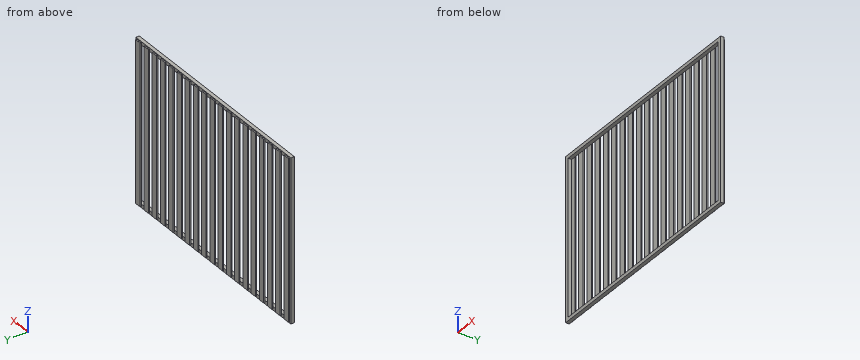
from build123d import *

# Parameters (mm, degrees)
F0_W     = 1900
F0_H     = 1400
F0_W_2   = 1840
F0_H_2   = 1340
F1_DEPTH = 15
F2_W     = 55
F2_H     = 10
F3_DEPTH = 690


# Not quite as in the source:
# - a feature names something its author has since deleted; it is built from what else it names


with BuildPart() as f1:
    # F0 (on Front) → F1 (new body, symmetric)
    with BuildSketch(Plane.XZ):
        Rectangle(F0_W, F0_H)
        Rectangle(F0_W_2, F0_H_2, mode=Mode.SUBTRACT)
    extrude(amount=F1_DEPTH, both=True)

    # F2 (on Top) → F3 (join, symmetric)
    with BuildSketch(Plane.XY):
        with Locations((-907.5, 20)):
            Rectangle(F2_W, F2_H)
        with Locations((-806.5, 20)):
            Rectangle(F2_W, F2_H)
        with Locations((-705.5, 20)):
            Rectangle(F2_W, F2_H)
        with Locations((-604.5, 20)):
            Rectangle(F2_W, F2_H)
        with Locations((-503.5, 20)):
            Rectangle(F2_W, F2_H)
        with Locations((-402.5, 20)):
            Rectangle(F2_W, F2_H)
        with Locations((-301.5, 20)):
            Rectangle(F2_W, F2_H)
        with Locations((-200.5, 20)):
            Rectangle(F2_W, F2_H)
        with Locations((-99.5, 20)):
            Rectangle(F2_W, F2_H)
        with Locations((1.5, 20)):
            Rectangle(F2_W, F2_H)
        with Locations((102.5, 20)):
            Rectangle(F2_W, F2_H)
        with Locations((203.5, 20)):
            Rectangle(F2_W, F2_H)
        with Locations((304.5, 20)):
            Rectangle(F2_W, F2_H)
        with Locations((405.5, 20)):
            Rectangle(F2_W, F2_H)
        with Locations((506.5, 20)):
            Rectangle(F2_W, F2_H)
        with Locations((607.5, 20)):
            Rectangle(F2_W, F2_H)
        with Locations((708.5, 20)):
            Rectangle(F2_W, F2_H)
        with Locations((809.5, 20)):
            Rectangle(F2_W, F2_H)
        with Locations((910.5, 20)):
            Rectangle(F2_W, F2_H)
    extrude(amount=F3_DEPTH, both=True)


solid = f1.part
Build history of the part. All positions in model axes, mm. Round coordinates to 2 decimals unless told otherwise and drop trailing zeros. Write each loop counter-clockwise with the first axis right and the second up, starting at its lowest first coordinate (ties: lowest second). Pieces come first, ordered by that corner, then holes. Notation, with made-up numbers: (43, 56.25) -> (53, 56.25) arc R24 ccw to (53, 88.25) -> close; hole circle Ø1 at (46, -13). An arc over 180 degrees is marked (long way). Write item = value, one per line.
(1) Flat gauge pins, fed straight in: pin 1 (3 mm diameter, centred on y = 22.5, z = -91, fed in from -X); pin 2 (8 mm diameter, centred on y = 20, z = 39, fed in from +X); pin 3 (3 mm diameter, centred on x = 600, y = 18, fed in from +Z); pin 4 (11 mm diameter, centred on x = -894.5, y = 19.5, fed in from +Z). Where does each tip first touch, or does it go through?
Answer:
pin_1 = -935
pin_2 = 938
pin_3 = 690
pin_4 = 700
(2) Band-saw the part on A-A (y = -1). Give the cut face in (x, z), then the cut area to 3 significant figures.
Answer:
outline = (-950, -700) -> (950, -700) -> (950, 700) -> (-950, 700) -> close; hole (-920, -670) -> (920, -670) -> (920, 670) -> (-920, 670) -> close
area = 194,000 mm2
(3) Probe L1, parallel to X at y = -1, z = 349; L2, parallel to Z at x = 377.5, y = -8; L3, parallel to Y at x = -327.5, z = -455. List the from-to ranges inside material, lowest first.
Answer:
L1 = -950 to -920, 920 to 950
L2 = -700 to -670, 670 to 700
L3 = 15 to 25
(4) Band-saw the part on B-B (z = -319). State how many separate pieces and enclosed holes the cut face has, then the cut area to 4 significant figures.
Answer:
separate_pieces = 19
enclosed_holes = 0
area = 12,250 mm2
